```python
from build123d import *

# Parameters (mm, degrees)
F1_DEPTH  = 15
F2_DEPTH  = 15
F3_R      = 10
F4_R      = 5
F5_R      = 3
F7_D      = 4.4
F8_R      = 4
F9_DEPTH  = 23.5
F10_W     = 15
F10_H     = 15
F11_DEPTH = 10
F12_DEPTH = 10
F10_R     = 1.65
F13_DEPTH = 15
F14_R     = 3


with BuildPart() as f1:
    # F0 (on Right) → F1 (new body)
    with BuildSketch(Plane.YZ):
        with BuildLine():
            Line((-50, 0), (0, 0))
            Line((0, 0), (50, 0))
            Line((50, 0), (50, 10))
            Line((50, 10), (6, 10))
            Line((6, 10), (0, 10))
            Line((0, 10), (-28, 10))
            ThreePointArc((-28, 10), (-35.0710678119, 12.9289321881), (-38, 20))
            Line((-38, 20), (-38, 48))
            Line((-38, 48), (-38, 54))
            Line((-38, 54), (-38, 110))
            Line((-38, 110), (-50, 110))
            Line((-50, 110), (-50, 10))
            Line((-50, 10), (-50, 0))
        make_face()
    extrude(amount=F1_DEPTH)

    # F0 (on Right) → F2 (join, through all)
    with BuildSketch(Plane.YZ):
        Polygon((0, 10), (6, 10), (-38, 54), (-38, 48), align=None)
    extrude(amount=F2_DEPTH)

    # F3
    f3_edges = [f1.edges().sort_by_distance(p)[0] for p in [
        (7.5, 6, 10),
        (7.5, -38, 54),
    ]]
    fillet(f3_edges, radius=F3_R)

    # F4
    f4_edges = [f1.edges().sort_by_distance(p)[0] for p in [
        (7.5, 0, 10),
        (7.5, -38, 48),
    ]]
    fillet(f4_edges, radius=F4_R)

    # F5
    f5_edges = [f1.edges().sort_by_distance(p)[0] for p in [
        (7.5, 50, 10),
        (7.5, -38, 110),
    ]]
    fillet(f5_edges, radius=F5_R)

    # F7 (through all)
    with Locations(Plane.XZ.offset(50)):
        with Locations((7.5, 100), (7.5, 25)):
            Hole(F7_D / 2)

    # F8 (on Front) → F9 (cut)
    with BuildSketch(Plane.XZ):
        with Locations((7.5, 25)):
            Circle(F8_R)
    extrude(amount=F9_DEPTH, mode=Mode.SUBTRACT)

    # F10 (on face) → F11 (join)
    with BuildSketch(Plane(origin=(0, 0, 0), x_dir=(1, 0, 0), z_dir=(0, 0, -1))):
        with Locations((7.5, 30.5)):
            Rectangle(F10_W, F10_H)
    extrude(amount=F11_DEPTH)

    # F10 (on face) → F12 (join)
    with BuildSketch(Plane(origin=(0, 0, 0), x_dir=(1, 0, 0), z_dir=(0, 0, -1))):
        with Locations((7.5, -30.5)):
            Rectangle(F10_W, F10_H)
    extrude(amount=F12_DEPTH)

    # F10 (on face) → F13 (cut)
    with BuildSketch(Plane(origin=(0, 0, 0), x_dir=(1, 0, 0), z_dir=(0, 0, -1))):
        with Locations((7.5, -42)):
            Circle(F10_R)
        with Locations((7.5, -18)):
            Circle(F10_R)
        with Locations((7.5, 44)):
            Circle(F10_R)
    extrude(amount=-F13_DEPTH, mode=Mode.SUBTRACT)

    # F14
    f14_edges = [f1.edges().sort_by_distance(p)[0] for p in [
        (15, -38, -5),
        (0, -38, -5),
        (0, -23, -5),
        (15, 23, -5),
        (15, 38, -5),
        (0, 38, -5),
        (0, 23, -5),
        (15, -23, -5),
    ]]
    fillet(f14_edges, radius=F14_R)


solid = f1.part
```
Input: part model. Units: mm. Frame: model coordinates. A direction names the side the tool comes from. Coordinates: 2 decimals unless noted, no trailing zeros. Loops run counter-clockwise (first coordinate to the right, second up) from the corner with the lowest first, then second, coordinate; pieces in that order, holes last. Notation, with made-up numbers: (82.5, 54) -> (129.5, 54) arc R30 cw to (129.5, 85) -> close; hole circle Ø4 at (-22.75, 88.25). An arc over 180 degrees is marked (long way). Use a Markdown table: item, result.
1) Pull-direction query (Z, two-part tool) for faces 6 (the cylindrical face through (7.605, -7.484, 13.011)), 7 (the flat face through (7, 50, 3)), 8 (the flat face through (7, 29, 10)); classes: released by +Z, released by -Z, zero draft, split by the parting line, or undercut.
Results found:
| item | result |
|---|---|
| face 6 | undercut |
| face 7 | zero draft |
| face 8 | released by +Z |
2) Cut plane B-B (y = 42). Return the cut outline in (x, z).
Results found:
| item | result |
|---|---|
| outline | (0, 0) -> (5.85, 0) -> (5.85, 10) -> (0, 10) -> close; (9.15, 0) -> (15, 0) -> (15, 10) -> (9.15, 10) -> close |
3) Access query for faces 1 (the cylindrical face through (0.86, -23.9, -5.07)), 2 (the flat face through (7, -38, 82)), 3 (the flat face through (7, -38, 28)), 4 (the cylindrical face through (14.1, 37.14, -5.07)), 5 (the flat face through (7, -23, -5)). Directions: +Z, -Z, +X, -X, +Y, -Y. A direction counts if a zero-diameter tool reaches every point of the face in a straight line with its end or side. Return the directions, or none.
Results found:
| item | result |
|---|---|
| face 1 | -Z, -X |
| face 2 | +Z, +X, -X, +Y |
| face 3 | +X, -X |
| face 4 | -Z, +X, +Y |
| face 5 | -Z, +X, -X |
4) Cut plane D-D (x = 7.5). Give the number of separate pieces and of enclosed holes in the cut face, then the cut area to 3 significant figures.
Results found:
| item | result |
|---|---|
| separate pieces | 5 |
| enclosed holes | 0 |
| area | 2,560 mm2 |
5) Cut plane A-A (z = 31). Return the cut outline in (x, y).
Results found:
| item | result |
|---|---|
| outline | (0, -50) -> (15, -50) -> (15, -38) -> (0, -38) -> close; (0, -21) -> (15, -21) -> (15, -15) -> (0, -15) -> close |
6) Material intervals for line 1 along Y through (x, z) = (7.5, 3.25); line 2 along X through (y, z) = (42, 2); line 3 along Y through (x, z) = (9, 64.5), sorted ascending. Write a range as from..to.
Results found:
| item | result |
|---|---|
| line 1 | y = -50..-45.65, -42.35..16.35, 19.65..40.35, 43.65..50 |
| line 2 | x = 0..5.85, 9.15..15 |
| line 3 | y = -50..-38 |
7) Contact query for flat-ended pins moving along their axis: pin 1 (1 mm diameter, centred on x = 8, y = -44.5, fed in from -Z); pin 2 (2.5 mm diameter, centred on x = 7.5, z = 100, fed in from -Y); pin 3 (4.5 mm diameter, centred on x = 7.5, y = 18, fed in from +Z); pin 4 (2.5 mm diameter, centred on x = 5.5, z = -3, fed in from -Y). Output: stop coordinate, or through.
Results found:
| item | result |
|---|---|
| pin 1 | stops at z = 15 |
| pin 2 | passes through |
| pin 3 | stops at z = 10 |
| pin 4 | stops at y = -38 |
8) Cut plane C-C (y = -44). Return the cut outline in (x, z), then the cut area to 3 significant figures.
Results found:
| item | result |
|---|---|
| outline | (0, 0) -> (5.85, 0) -> (5.85, 15) -> (9.15, 15) -> (9.15, 0) -> (15, 0) -> (15, 110) -> (0, 110) -> close; hole circle Ø4.4 at (7.5, 25); hole circle Ø4.4 at (7.5, 100) |
| area | 1,570 mm2 |
